The model under review builds one solid part; all positions refer to its coordinate system, in mm. A direction names the side the tool comes from. Coordinates: 2 decimals unless noted, no trailing zeros. Order: outer loops, then holes, each group sorted by start corner. A loop starts at its lowest first (then second) coordinate and runs counter-clockwise, first axis right, second up. Notation, with made-up numbers: M 68.25,88.25 L 102.25,88.25 A18 cw 102.25,104.25 Z; hole C -9.5,-6.75 d7. An arc over 180 degrees is marked long. Answer in a Markdown table with one row per item.
from build123d import *

# Parameters (mm, degrees)
SKETCH1_R                 = 7.8232
BOSS_EXTRUDE1_DEPTH       = 0.8636
SKETCH2_R                 = 2.6289
BOSS_EXTRUDE2_DEPTH       = 6.2738
TAP_DRILL_FOR_8_32_TAP1_D = 3.4544


with BuildPart() as part:
    # Sketch1 → Boss-Extrude1 (new body)
    with BuildSketch(Plane.XY):
        Circle(SKETCH1_R)
    extrude(amount=BOSS_EXTRUDE1_DEPTH)

    # Sketch2 → Boss-Extrude2 (add)
    with BuildSketch(Plane.XY.offset(0.8636)):
        with Locations(Location((0, 0, 0), (0, 0, 180))):
            Circle(SKETCH2_R)
    extrude(amount=BOSS_EXTRUDE2_DEPTH)

    # Tap Drill for #8-32 Tap1 (through all)
    with Locations(Plane.XY.offset(7.1374)):
        with Locations((0, 0)):
            Hole(TAP_DRILL_FOR_8_32_TAP1_D / 2)


solid = part.part
(1) Take a section at D-D (x = 2). Write out the cut boundary in (y, z).
Report:
| item | result |
|---|---|
| outline | M -7.56,0 L 7.56,0 L 7.56,0.86 L 1.71,0.86 L 1.71,7.14 L -1.71,7.14 L -1.71,0.86 L -7.56,0.86 Z |
(2) Machinability: for faces 1 (the flat face through (-1, 2, 7.137)), 2 (the cylindrical face through (-2.508, -0.79, 3.957)), which of the approach directions +Z, -Z, +X, -X, +Y, -Y give a long, thin tool a straight path to every point of the face, cutting with its end or side? Answer none if there is none.
Report:
| item | result |
|---|---|
| face 1 | +Z, +X, -X, +Y, -Y |
| face 2 | +Z |
(3) Insertion check: P1, Ø1, axis at x = 1, z = 2, coming from the -Y side; P2, Ø4, axis at x = 3, y = -0.5, coming from the +Z side; P3, Ø1, axis at x = 3.5, z = 1, coming from the -Y side; P4, Ø1, axis at y = -2, z = 5, coming from the -X side. Each pin has a flat end and moves straight along its axis. Give the tip position at first contact, or say it passes through.
Report:
| item | result |
|---|---|
| P1 | y = -2.58 |
| P2 | z = 7.14 |
| P3 | y = -7.22 |
| P4 | x = -2.16 |
(4) Take a section at A-A (y = 0). Write out the cut boundary in (x, z).
Report:
| item | result |
|---|---|
| outline | M -7.82,0 L -1.73,0 L -1.73,7.14 L -2.63,7.14 L -2.63,0.86 L -7.82,0.86 Z; M 1.73,0 L 7.82,0 L 7.82,0.86 L 2.63,0.86 L 2.63,7.14 L 1.73,7.14 Z |
(5) The part is to be moulded in two halves that separate along Y. For faces 3 (the cylindrical face through (0.225, 1.713, 3.519)), 4 (the cylindrical face through (7.46, 2.35, 0.43)), 5 (the flat face through (0, 2, 0)), say which applies: +Y half, -Y half, draft (parallel to the pull), parting line (faces both ways), or undercut.
Report:
| item | result |
|---|---|
| face 3 | undercut |
| face 4 | parting line |
| face 5 | draft |
(6) To check wall thickness, follow line 1 (Y direction, x = 0, z = 2.5); line 2 (Z direction, x = -1, y = 5.25); line 3 (Y direction, x = 2.25, z = 3.25). State the ranges of each line that lie inside material, in increasing order. Write a range as [from, to].
Report:
| item | result |
|---|---|
| line 1 | [-2.63, -1.73], [1.73, 2.63] |
| line 2 | [0, 0.86] |
| line 3 | [-1.36, 1.36] |
(7) Take a section at C-C (z = 1.5). Write out the cut boundary in (x, y).
Report:
| item | result |
|---|---|
| outline | C 0,0 d5.26; hole C 0,0 d3.45 |
